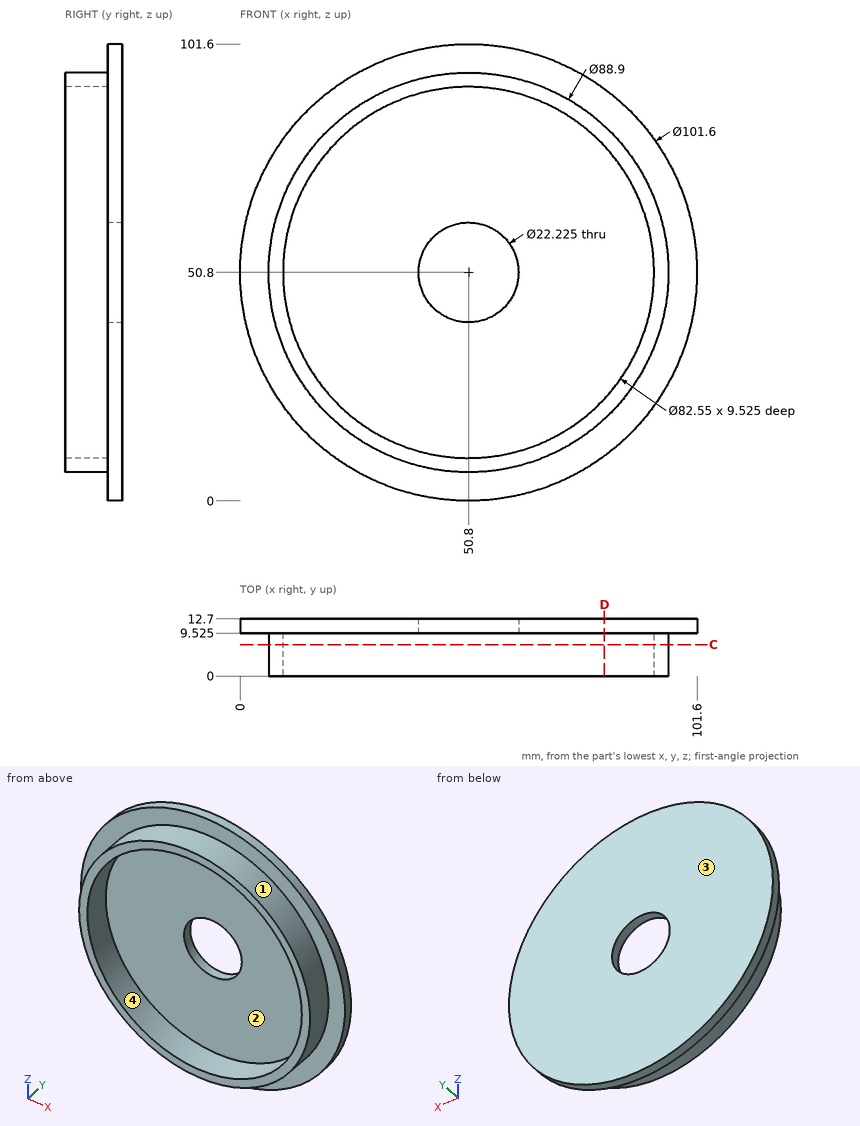
The figure shows three views and two pictorial views of one solid part (mm, origin at its lowest corner). Answer the questions. Give positions to 0.01 mm unless a question says otherwise; leave off trailing zeros. Write each loop counter-clockwise with the first axis right and the second up, starting at its lowest first coordinate (ties: lowest second). Pieces come first, ordered by that corner, then holes. Notation, with made-up numbers: (-5.5, 28) - (29.5, 28) arc R20 ccw to (29.5, 64) - close; hole circle Ø9 at (70.25, -24.75). An arc over 180 degrees is marked (long way). Use one line per item in the form item = value. Start each with the question number.
1) The mould has two halves that part along X. Classify the marked faces 1, 2, 3 and 4: pulls with the +X half, pulls with the -X half, needs draft (parallel to the pull), parting line crosses it, or undercut.
2) Find section D-D on x = 81. Determine the outline of the cut face in (y, z) (1 decimal), plus the area to 3 significant figures.
3) Find section C-C on y = 7. Determine the outline of the cut face in (x, z) (3 decimals), plus the area to 3 significant figures.
4) Flat-ended cylindrical pins translate along their axes: pin 1 Ø3 at (y, z) = (2, 16) entering from +X; pin 2 Ø1.5 at (y, z) = (3, 30) entering from +X; pin 3 Ø18 at (x, z) = (50.8, 50.8) entering from -Y; pin 4 Ø5 at (x, y) = (78.5, 5) entering from -Z. Find the tip coordinate at first contact, or state that the pin passes through.
5) Consider line 1 along Z through (x, y) = (50.8, 3) (3 decimals); line 2 along Y through (x, z) = (76, 58) (3 decimals); line 3 along Z through (x, y) = (17, 7.75). Determine where each line is inside the solid, lowest interval first. Write a range as from..to.
Geometry results:
q1.face_1 = parting line crosses it
q1.face_2 = undercut
q1.face_3 = needs draft
q1.face_4 = undercut
q2.outline = (0, 18.2) - (9.5, 18.2) - (9.5, 10) - (12.7, 10) - (12.7, 91.6) - (9.5, 91.6) - (9.5, 83.4) - (0, 83.4) - (0, 78.9) - (9.5, 78.9) - (9.5, 22.7) - (0, 22.7) - close
q2.area = 345 mm2
q3.outline = circle Ø88.9 at (50.8, 50.8); hole circle Ø82.55 at (50.8, 50.8)
q3.area = 855 mm2
q4.pin_1 = 80.24
q4.pin_2 = 90.47
q4.pin_3 = through
q4.pin_4 = 14.18
q5.line_1 = 6.35..9.525, 92.075..95.25
q5.line_2 = 9.525..12.7
q5.line_3 = 21.93..27.11, 74.49..79.67
